from build123d import *

# Parameters (mm, degrees)
F4_R            = 3.5
F5_DEPTH        = 4
F6_D            = 2.5
F6_CBORE_D      = 4.5
F6_CBORE_DEPTH  = 2
F7_DEPTH        = 20
F9_D            = 2.9
F9_DEPTH        = 18
F9_CSINK_D      = 4
F9_CSINK_ANGLE  = 90
F9_TIP          = 0.8712478976
F11_D           = 2.9
F11_DEPTH       = 18
F11_CSINK_D     = 4
F11_CSINK_ANGLE = 90
F11_TIP         = 0.8712478976
F13_D           = 2.9
F13_DEPTH       = 18
F13_CSINK_D     = 4
F13_CSINK_ANGLE = 90
F13_TIP         = 0.8712478976
F15_D           = 2.9
F15_DEPTH       = 18
F15_CSINK_D     = 4
F15_CSINK_ANGLE = 90
F15_TIP         = 0.8712478976
F16_DEPTH       = 25
F18_DEPTH       = 25
F19_DEPTH       = 25
F20_W           = 20
F20_H           = 30.4843550548
F20_H_2         = 31.25
F20_H_3         = 30.620081059
F21_DEPTH       = 4
F17_R           = 7.5
F22_DEPTH       = 4
F23_W           = 43
F23_H           = 4
F24_DEPTH       = 10
F26_D           = 2.5
F26_DEPTH       = 15
F26_CSINK_D     = 4
F26_CSINK_ANGLE = 90
F26_TIP         = 0.7510757738
F27_D           = 2.5
F27_DEPTH       = 15
F27_CSINK_D     = 4
F27_CSINK_ANGLE = 90
F27_TIP         = 0.7510757738


with BuildPart() as f5:
    # F4 (on Top) → F5 (new body)
    with BuildSketch(Plane.XY):
        Polygon((27.5709562153, 77.495081059), (-22.4290437847, 77.495081059), (-22.4290437847, 73.495081059), (-22.4290437847, -18.5049188996), (-22.4290437847, -22.504918941), (27.5709562153, -22.504918941), (27.5709562153, -18.504918941), (27.5709562153, 73.495081059), align=None)
        with BuildLine():
            ThreePointArc((-15.4290437847, -18.504918941), (-18.9290438054, -22.004918941), (-22.4290437847, -18.5049188996))
            ThreePointArc((-22.4290437847, -18.5049188996), (-18.9290437641, -15.004918941), (-15.4290437847, -18.504918941))
        make_face(mode=Mode.SUBTRACT)
        with Locations((24.0709562153, -18.504918941)):
            Circle(F4_R, mode=Mode.SUBTRACT)
        with BuildLine():
            Line((-3.6008084906, 42.745081059), (-14.6290437847, 69.995081059))
            Line((-14.6290437847, 69.995081059), (-0.6790437847, 69.995081059))
            ThreePointArc((-0.6790437847, 69.995081059), (2.5709562153, 73.245081059), (5.8209562153, 69.995081059))
            Line((5.8209562153, 69.995081059), (19.7709562153, 69.995081059))
            Line((19.7709562153, 69.995081059), (8.7427209211, 42.745081059))
            Line((8.7427209211, 42.745081059), (16.0709562153, 42.745081059))
            ThreePointArc((16.0709562153, 42.745081059), (17.8209562153, 44.495081059), (19.5709562153, 42.745081059))
            ThreePointArc((19.5709562153, 42.745081059), (19.0583930823, 41.507644192), (17.8209562153, 40.995081059))
            Line((17.8209562153, 40.995081059), (17.8209562153, 13.995081059))
            ThreePointArc((17.8209562153, 13.995081059), (19.0583930823, 13.4825179261), (19.5709562153, 12.245081059))
            ThreePointArc((19.5709562153, 12.245081059), (17.8209562153, 10.495081059), (16.0709562153, 12.245081059))
            Line((16.0709562153, 12.245081059), (8.7427209211, 12.245081059))
            Line((8.7427209211, 12.245081059), (-3.6008084906, 12.245081059))
            Line((-3.6008084906, 12.245081059), (-10.9290437847, 12.245081059))
            ThreePointArc((-10.9290437847, 12.245081059), (-13.9164806518, 11.007644192), (-12.6790437847, 13.995081059))
            Line((-12.6790437847, 13.995081059), (-12.6790437847, 40.995081059))
            ThreePointArc((-12.6790437847, 40.995081059), (-13.9164806518, 43.9825179261), (-10.9290437847, 42.745081059))
            Line((-10.9290437847, 42.745081059), (-3.6008084906, 42.745081059))
        make_face(mode=Mode.SUBTRACT)
        with BuildLine():
            ThreePointArc((-15.4290437847, 73.495081059), (-18.9290437847, 69.995081059), (-22.4290437847, 73.495081059))
            ThreePointArc((-22.4290437847, 73.495081059), (-18.9290437847, 76.995081059), (-15.4290437847, 73.495081059))
        make_face(mode=Mode.SUBTRACT)
        with Locations((24.0709562153, 73.495081059)):
            Circle(F4_R, mode=Mode.SUBTRACT)
        with BuildLine():
            ThreePointArc((-15.4290437847, -18.504918941), (-18.9290437641, -15.004918941), (-22.4290437847, -18.5049188996))
            ThreePointArc((-22.4290437847, -18.5049188996), (-18.9290438054, -22.004918941), (-15.4290437847, -18.504918941))
        make_face()
        with Locations((24.0709562153, -18.504918941)):
            Circle(F4_R)
        with BuildLine():
            ThreePointArc((-15.4290437847, 73.495081059), (-18.9290437847, 76.995081059), (-22.4290437847, 73.495081059))
            ThreePointArc((-22.4290437847, 73.495081059), (-18.9290437847, 69.995081059), (-15.4290437847, 73.495081059))
        make_face()
        with Locations((24.0709562153, 73.495081059)):
            Circle(F4_R)
        with BuildLine():
            Line((8.7427209211, 42.745081059), (2.5709562153, 27.495081059))
            Line((2.5709562153, 27.495081059), (8.7427209211, 12.245081059))
            Line((8.7427209211, 12.245081059), (16.0709562153, 12.245081059))
            ThreePointArc((16.0709562153, 12.245081059), (16.5835193482, 13.4825179261), (17.8209562153, 13.995081059))
            Line((17.8209562153, 13.995081059), (17.8209562153, 40.995081059))
            ThreePointArc((17.8209562153, 40.995081059), (16.5835193482, 41.507644192), (16.0709562153, 42.745081059))
            Line((16.0709562153, 42.745081059), (8.7427209211, 42.745081059))
        make_face()
        with BuildLine():
            Line((2.5709562153, 27.495081059), (-3.6008084906, 42.745081059))
            Line((-3.6008084906, 42.745081059), (-10.9290437847, 42.745081059))
            ThreePointArc((-10.9290437847, 42.745081059), (-11.4416069177, 41.507644192), (-12.6790437847, 40.995081059))
            Line((-12.6790437847, 40.995081059), (-12.6790437847, 13.995081059))
            ThreePointArc((-12.6790437847, 13.995081059), (-11.4416069177, 13.4825179261), (-10.9290437847, 12.245081059))
            Line((-10.9290437847, 12.245081059), (-3.6008084906, 12.245081059))
            Line((-3.6008084906, 12.245081059), (2.5709562153, 27.495081059))
        make_face()
        Polygon((8.7427209211, 42.745081059), (-3.6008084906, 42.745081059), (2.5709562153, 27.495081059), align=None)
        Polygon((8.7427209211, 12.245081059), (2.5709562153, 27.495081059), (-3.6008084906, 12.245081059), align=None)
        with BuildLine():
            Line((-0.6790437847, 69.995081059), (-14.6290437847, 69.995081059))
            Line((-14.6290437847, 69.995081059), (-3.6008084906, 42.745081059))
            Line((-3.6008084906, 42.745081059), (8.7427209211, 42.745081059))
            Line((8.7427209211, 42.745081059), (19.7709562153, 69.995081059))
            Line((19.7709562153, 69.995081059), (5.8209562153, 69.995081059))
            ThreePointArc((5.8209562153, 69.995081059), (2.5709562153, 66.745081059), (-0.6790437847, 69.995081059))
        make_face()
    extrude(amount=F5_DEPTH)

    # F6 (through all)
    with Locations(Plane(origin=(0, 0, 0), x_dir=(1, 0, 0), z_dir=(0, 0, -1))):
        with Locations((19.7709562153, -69.995081059), (19.7709562153, 15.004918941), (-14.6290437847, 15.004918941), (-14.6290437847, -69.995081059)):
            CounterBoreHole(F6_D / 2, F6_CBORE_D / 2, F6_CBORE_DEPTH)

    # F4 (on Top) → F7 (join)
    with BuildSketch(Plane.XY):
        with BuildLine():
            ThreePointArc((-15.4290437847, -18.504918941), (-18.9290437641, -15.004918941), (-22.4290437847, -18.5049188996))
            ThreePointArc((-22.4290437847, -18.5049188996), (-18.9290438054, -22.004918941), (-15.4290437847, -18.504918941))
        make_face()
        with Locations((24.0709562153, -18.504918941)):
            Circle(F4_R)
        with BuildLine():
            ThreePointArc((-15.4290437847, 73.495081059), (-18.9290437847, 76.995081059), (-22.4290437847, 73.495081059))
            ThreePointArc((-22.4290437847, 73.495081059), (-18.9290437847, 69.995081059), (-15.4290437847, 73.495081059))
        make_face()
        with Locations((24.0709562153, 73.495081059)):
            Circle(F4_R)
    extrude(amount=-F7_DEPTH)

    # F9
    with Locations(Plane(origin=(0, 0, -20), x_dir=(1, 0, 0), z_dir=(0, 0, -1))):
        with Locations((-18.9290437847, -73.495081059)):
            CounterSinkHole(F9_D / 2, F9_CSINK_D / 2, depth=F9_DEPTH, counter_sink_angle=F9_CSINK_ANGLE)
            with Locations((0, 0, -(F9_DEPTH + F9_TIP / 2))):  # 118° drill point
                Cone(0, F9_D / 2, F9_TIP, mode=Mode.SUBTRACT)

    # F11
    with Locations(Plane(origin=(0, 0, -20), x_dir=(1, 0, 0), z_dir=(0, 0, -1))):
        with Locations((-18.9290437847, 18.504918941)):
            CounterSinkHole(F11_D / 2, F11_CSINK_D / 2, depth=F11_DEPTH, counter_sink_angle=F11_CSINK_ANGLE)
            with Locations((0, 0, -(F11_DEPTH + F11_TIP / 2))):  # 118° drill point
                Cone(0, F11_D / 2, F11_TIP, mode=Mode.SUBTRACT)

    # F13
    with Locations(Plane(origin=(0, 0, -20), x_dir=(1, 0, 0), z_dir=(0, 0, -1))):
        with Locations((24.0709562153, -73.495081059)):
            CounterSinkHole(F13_D / 2, F13_CSINK_D / 2, depth=F13_DEPTH, counter_sink_angle=F13_CSINK_ANGLE)
            with Locations((0, 0, -(F13_DEPTH + F13_TIP / 2))):  # 118° drill point
                Cone(0, F13_D / 2, F13_TIP, mode=Mode.SUBTRACT)

    # F15
    with Locations(Plane(origin=(0, 0, -20), x_dir=(1, 0, 0), z_dir=(0, 0, -1))):
        with Locations((24.0709562153, 18.504918941)):
            CounterSinkHole(F15_D / 2, F15_CSINK_D / 2, depth=F15_DEPTH, counter_sink_angle=F15_CSINK_ANGLE)
            with Locations((0, 0, -(F15_DEPTH + F15_TIP / 2))):  # 118° drill point
                Cone(0, F15_D / 2, F15_TIP, mode=Mode.SUBTRACT)

    # F16 (add): a face of the model
    f16_faces = [f5.faces().sort_by_distance(p)[0] for p in [
        (2.5709562153, -22.504918941, 2),
    ]]
    extrude(f16_faces, amount=F16_DEPTH)

    # F18 (add): a face of the model
    f18_faces = [f5.faces().sort_by_distance(p)[0] for p in [
        (27.5709562153, 14.995081059, 2),
    ]]
    extrude(f18_faces, amount=F18_DEPTH)

    # F19 (add): a face of the model
    f19_faces = [f5.faces().sort_by_distance(p)[0] for p in [
        (-22.4290437847, 14.995081059, 2),
    ]]
    extrude(f19_faces, amount=F19_DEPTH)

    # F20 (on face) → F21 (cut)
    with BuildSketch(Plane.XY.offset(4)):
        with Locations((-32.4290437847, -23.6845964684)):
            Rectangle(F20_W, F20_H)
        with Locations((-32.4290437847, 14.995081059)):
            Rectangle(F20_W, F20_H_2)
        with Locations((-32.4290437847, 54.057581059)):
            Rectangle(F20_W, F20_H_2)
        with Locations((37.5709562153, 54.057581059)):
            Rectangle(F20_W, F20_H_2)
        with Locations((37.5709562153, 15.3100405295)):
            Rectangle(F20_W, F20_H_3)
        with Locations((37.5709562153, -24.067418941)):
            Rectangle(F20_W, F20_H_2)
    extrude(amount=-F21_DEPTH, mode=Mode.SUBTRACT)

    # F17 (on face) → F22 (cut)
    with BuildSketch(Plane.XY.offset(4)):
        with Locations((-7.4290437847, -32.2756583249)):
            Circle(F17_R)
        with Locations((12.5709562153, -32.2756583249)):
            Circle(F17_R)
    extrude(amount=-F22_DEPTH, mode=Mode.SUBTRACT)

    # F23 (on face) → F24 (join)
    with BuildSketch(Plane.XZ.offset(47.504918941)):
        with Locations((2.5709562153, 2)):
            Rectangle(F23_W, F23_H)
    extrude(amount=F24_DEPTH)

    # F26
    with Locations(Plane(origin=(0, 0, 0), x_dir=(1, 0, 0), z_dir=(0, 0, -1))):
        with Locations((2.5709562153, 52.504918941), (2.5709562153, 42.504918941)):
            CounterSinkHole(F26_D / 2, F26_CSINK_D / 2, depth=F26_DEPTH, counter_sink_angle=F26_CSINK_ANGLE)
            with Locations((0, 0, -(F26_DEPTH + F26_TIP / 2))):  # 118° drill point
                Cone(0, F26_D / 2, F26_TIP, mode=Mode.SUBTRACT)

    # F27
    with Locations(Plane(origin=(0, 0, 0), x_dir=(1, 0, 0), z_dir=(0, 0, -1))):
        with Locations((-18.9290437847, 42.504918941), (-18.9290437847, 32.504918941), (24.0709562153, 32.504918941), (24.0709562153, 42.504918941)):
            CounterSinkHole(F27_D / 2, F27_CSINK_D / 2, depth=F27_DEPTH, counter_sink_angle=F27_CSINK_ANGLE)
            with Locations((0, 0, -(F27_DEPTH + F27_TIP / 2))):  # 118° drill point
                Cone(0, F27_D / 2, F27_TIP, mode=Mode.SUBTRACT)


solid = f5.part
Here's how the part is built. I have some questions about the finished solid (model axes, mm). A direction names the side the tool comes from. Give positions to 0.01 mm unless a question says otherwise; leave off trailing zeros. Loops run counter-clockwise (first coordinate to the right, second up) from the corner with the lowest first, then second, coordinate; pieces in that order, holes last. Notation, with made-up numbers: (2.25, 49) -> (21.25, 49) arc R15 cw to (21.25, 62) -> close; hole circle Ø4 at (44, 9.5). An arc over 180 degrees is marked (long way). Answer as a JSON object with one key per item and string values. Group by question number.
Item 1: Imagine slicing it at D-D on x = -6.5. Write out the boundary of the cut face in (y, z).
Item 2: I need wall thicknesses on L1, parallel to Y at x = 40.5, z = 1.25; L2, parallel to Y at x = -33.5, z = 2.5; L3, parallel to Z at x = -16.5, y = 39. Which ranges of each line are inside material? Lowest first, please.
Item 3: Thinking about a two-plate mould opening in X: for faces 1 (the cylindrical face through (27.41, -17.45, -9.86)), 2 (the flat face through (-18.929, -52, 2)), 3 (the flat face through (-17, -20, -20)), which applies, pulls with the +X half, pulls with the -X half, needs draft (parallel to the pull), parting line crosses it, or undercut?
Item 4: On a 3-axis mill with a long thin cutter (end or side, diameter ignored), from which of +Z, -Z, +X, -X, +Y, -Y can I reach the whole of each face in a straight line? I mean faces 4 (the flat face through (39, -47.505, 2)), 5 (the cylindrical face through (27.41, 74.55, -9.86)), 6 (the flat face through (37, -39.692, 2)). Say none if no direction works.
Item 5: Imagine slicing it at C-C on y = 58.5. Write out the boundary of the cut face in (x, z).
Item 6: Imagine slicing it at B-B on x = 35. Write out the boundary of the cut face in (y, z), then the cut area to 3 significant figures.
Item 7: Will these pins go through, and if not, where does the flat tip stop? pin 1 (2 mm diameter, centred on x = -28.5, z = 1, fed in from -Y); pin 2 (3.5 mm diameter, centred on x = 19.77, y = -15, fed in from -Z); pin 3 (12 mm diameter, centred on x = 19, z = -8.5, fed in from +Y); pin 4 (12 mm diameter, centred on x = 6, z = -4.5, fed in from +Y).
Item 8: Imagine slicing it at A-A on z = -13.25. Write out the boundary of the cut face in (x, y).
Answer list:
{
 "1": {"outline": "(-57.5, 0) -> (-39.72, 0) -> (-39.72, 4) -> (-57.5, 4) -> close; (-24.83, 0) -> (77.5, 0) -> (77.5, 4) -> (-24.83, 4) -> close"},
 "2": {"L1": "y = -47.5 to -39.69, -8.44 to 0, 30.62 to 38.43, 69.68 to 77.5", "L2": "y = -47.5 to -38.93, -8.44 to -0.63, 30.62 to 38.43, 69.68 to 77.5", "L3": "z = 0 to 4"},
 "3": {"face 1": "undercut", "face 2": "pulls with the -X half", "face 3": "needs draft"},
 "4": {"face 4": "+Z, -Z, +X, -Y", "face 5": "-Z", "face 6": "+Z, -Z"},
 "5": {"outline": "(-47.43, 0) -> (-42.43, 0) -> (-42.43, 4) -> (-47.43, 4) -> close; (-22.43, 0) -> (27.57, 0) -> (27.57, 4) -> (-22.43, 4) -> close; (47.57, 0) -> (52.57, 0) -> (52.57, 4) -> (47.57, 4) -> close"},
 "6": {"outline": "(-47.5, 0) -> (-39.69, 0) -> (-39.69, 4) -> (-47.5, 4) -> close; (-8.44, 0) -> (0, 0) -> (0, 4) -> (-8.44, 4) -> close; (30.62, 0) -> (38.43, 0) -> (38.43, 4) -> (30.62, 4) -> close; (69.68, 0) -> (77.5, 0) -> (77.5, 4) -> (69.68, 4) -> close", "area": "128 mm2"},
 "7": {"pin 1": "stops at y = -47.5", "pin 2": "stops at z = 2", "pin 3": "stops at y = 77", "pin 4": "stops at y = 77.5"},
 "8": {"outline": "circle Ø7 at (-18.93, -18.5); circle Ø7 at (-18.93, 73.5); circle Ø7 at (24.07, -18.5); circle Ø7 at (24.07, 73.5); hole circle Ø2.9 at (-18.93, -18.5); hole circle Ø2.9 at (-18.93, 73.5); hole circle Ø2.9 at (24.07, -18.5); hole circle Ø2.9 at (24.07, 73.5)"}
}
